```python
from build123d import *

# Parameters (mm, degrees)
F0_R     = 20
F1_DEPTH = 80
F2_T     = -4
F3_R     = 17.798556
F4_DEPTH = 5.2


with BuildPart() as f1:
    # F0 (on Front) → F1 (new body)
    with BuildSketch(Plane.XZ):
        Circle(F0_R)
    extrude(amount=F1_DEPTH)

    # F2
    f2_openings = [f1.faces().sort_by_distance(p)[0] for p in [
        (0, -80, 0),
    ]]
    offset(amount=F2_T, openings=f2_openings)

    # F3 (on face) → F4 (cut)
    with BuildSketch(Plane.XZ.offset(80)):
        Circle(F3_R)
    extrude(amount=-F4_DEPTH, mode=Mode.SUBTRACT)


solid = f1.part
```
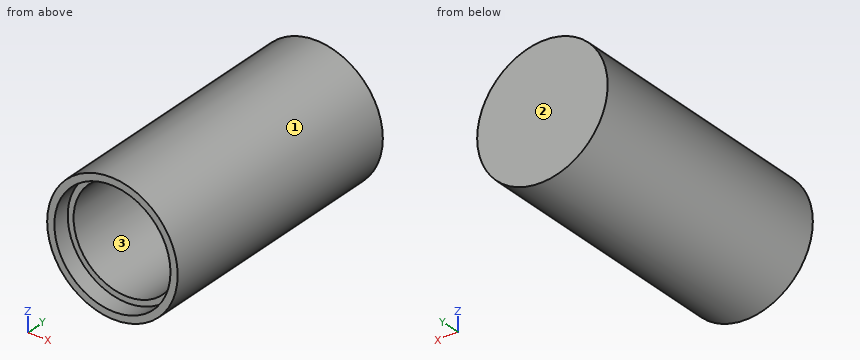
Geometry check sheet. Reference: the model listing, model coordinates, mm. Face numbers are marked on the shaded views. Give positions to 0.01 mm unless a question says otherwise; leave off trailing zeros. Write each loop counter-clockwise with the first axis right and the second up, starting at its lowest first coordinate (ties: lowest second). Pieces come first, ordered by that corner, then holes.
1) Section check A-A, the plane x = 0. Record the boundary of the cut face in (y, z).
2) Section check C-C, the plane z = -11. Record the boundary of the cut face in (x, y).
3) Material ranges on L1, parallel to Z at x = 0, y = -47; L2, parallel to Z at x = 0, y = -77.55; L3, parallel to Y at x = -14.5, z = -3.5, recorded low to high.
4) Release check for a two-part mould opening along X. For the marked faces 1, 2 and 3 record: pulls with the +X half, pulls with the -X half, needs draft (parallel to the pull), parting line crosses it, or undercut.
5) Gauge pin test, flat ends, axial feed: pin 1 (1 mm diameter, centred on y = -41.5, z = -2.5, fed in from -X); pin 2 (16 mm diameter, centred on x = -1.5, z = 3, fed in from -Y); pin 3 (3 mm diameter, centred on y = -59, z = 13, fed in from +X). Record the tip position at first contact, or that the pin passes through.
6) Section check B-B, the plane y = -15. Record the boundary of the cut face in (x, z).
Computed:
1. outline: (-80, -20) - (0, -20) - (0, 20) - (-80, 20) - (-80, 17.8) - (-74.8, 17.8) - (-74.8, 16) - (-4, 16) - (-4, -16) - (-74.8, -16) - (-74.8, -17.8) - (-80, -17.8) - close
2. outline: (-16.7, -80) - (-13.99, -80) - (-13.99, -74.8) - (-11.62, -74.8) - (-11.62, -4) - (11.62, -4) - (11.62, -74.8) - (13.99, -74.8) - (13.99, -80) - (16.7, -80) - (16.7, 0) - (-16.7, 0) - close
3. L1: z = -20 to -16, 16 to 20
3. L2: z = -20 to -17.8, 17.8 to 20
3. L3: y = -4 to 0
4. face 1: parting line crosses it
4. face 2: needs draft
4. face 3: undercut
5. pin 1: stops at x = -19.9
5. pin 2: stops at y = -4
5. pin 3: stops at x = 16.36
6. outline: circle Ø40 at (0, 0); hole circle Ø32 at (0, 0)
